Answer from the drawing. Dimensions are ordinates in mm from the lowest x, y and z of the part. A direction names the side the tool comes from. Coordinates: 2 decimals unless noted, no trailing zeros. Order: outer loops, then holes, each group sorted by start corner. A loop starts at its lowest first (then second) coordinate and runs counter-clockwise, first axis right, second up. Notation, with made-up numbers: M 18,1.5 L 73,1.5 A14 ccw 73,13.5 Z; hole C 24.25,84.25 d11. An arc over 180 degrees is marked long. Use a Markdown table: item, result.
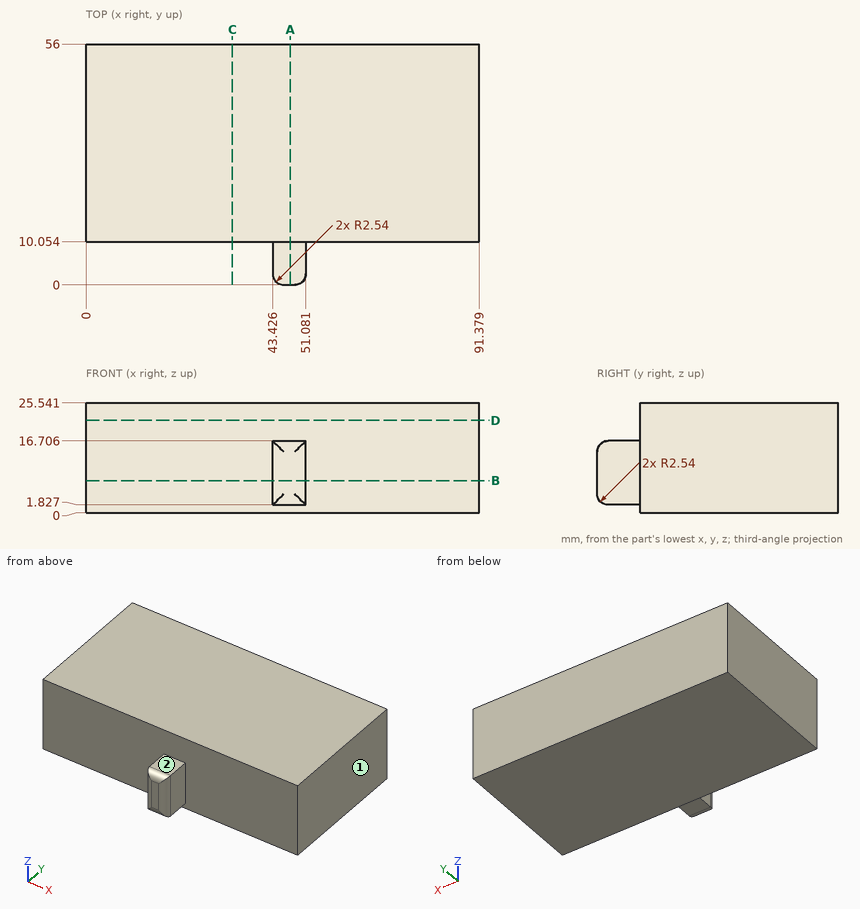
(1) A cutting plane is placed at A-A (x = 47.5). Determine the outline of the cut face in (y, z) (1 decimal), then the cut area to 3 significant figures.
Conclusion:
| item | result |
|---|---|
| outline | M 0,4.4 A2.5 ccw 2.5,1.8 L 10.1,1.8 L 10.1,0 L 56,0 L 56,25.5 L 10.1,25.5 L 10.1,16.7 L 2.5,16.7 A2.5 ccw 0,14.2 Z |
| area | 1,320 mm2 |
(2) A cutting plane is placed at B-B (z = 7.5). Determine the outline of the cut face in (x, y) (1 decimal).
Conclusion:
| item | result |
|---|---|
| outline | M 0,10.1 L 43.4,10.1 L 43.4,2.5 A2.5 ccw 46,0 L 48.5,0 A2.5 ccw 51.1,2.5 L 51.1,10.1 L 91.4,10.1 L 91.4,56 L 0,56 Z |
(3) A cutting plane is placed at C-C (x = 34). Determine the outline of the cut face in (y, z) (1 decimal).
Conclusion:
| item | result |
|---|---|
| outline | M 10.1,0 L 56,0 L 56,25.5 L 10.1,25.5 Z |
(4) A cutting plane is placed at D-D (z = 21.5). Determine the outline of the cut face in (x, y) (1 decimal), then the cut area to 3 significant figures.
Conclusion:
| item | result |
|---|---|
| outline | M 0,10.1 L 91.4,10.1 L 91.4,56 L 0,56 Z |
| area | 4,200 mm2 |
(5) Straight lines are drawn through the part: L1, parallel to Y at x = 8, z = 17.75 (1 decimal); L2, parallel to Y at x = 45, z = 15. For each, find the intervals that lie inside material, in ascending order.
Conclusion:
| item | result |
|---|---|
| L1 | 10.1 to 56 |
| L2 | 0.19 to 56 |
(6) Given P1, Ø13, axis at x = 45, z = 9.5, coming from the -Y side; P2, Ø6, axis at x = 48, y = 5.5, coming from the +Z side; P3, Ø4, axis at y = 5, z = 8, coming from the +X side; P4, Ø3, axis at x = 33.5, z = 5.5, coming from the -Y side, each flat-ended and moving along its own axis, determine where each tip first touches the part or whether it passes through.
Conclusion:
| item | result |
|---|---|
| P1 | y = 0 |
| P2 | z = 16.71 |
| P3 | x = 51.08 |
| P4 | y = 10.05 |
(7) Which of the six approach directions +Z, -Z, +X, -X, +Y, -Y give full straight-line access (tool end or side, diameter ignored) to the marked faces 1 and 2?
Conclusion:
| item | result |
|---|---|
| face 1 | +Z, -Z, +X, +Y, -Y |
| face 2 | +Z, +X, -X, -Y |
